The model under review builds one solid part; all positions refer to its coordinate system, in mm. Face numbers are marked on the shaded views. A direction names the side the tool comes from. Round coordinates to 2 decimals unless told otherwise and drop trailing zeros. Write each loop counter-clockwise with the first axis right and the second up, starting at its lowest first coordinate (ties: lowest second). Pieces come first, ordered by that corner, then holes. Notation, with made-up numbers: M 40.5,-32 L 84.5,-32 A10 cw 84.5,-20 Z; hole C 17.5,-37 d11. An arc over 180 degrees is marked long. One line per item, written item: value. Start each with the question number.
1) Wall thickness on probe 1 along Z at (x, y) = (-5.75, -1.95); probe 2 along X at (y, z) = (-2.05, -0.25); probe 3 along Z at (x, y) = (5.25, -2.4): over which ranges is each line inside the solid? List them lowest first.
2) Mouldability with a two-part tool opening along Z and no side actions: class the marked faces 4, 5 and 6 as +Z half, -Z half, draft (parallel to the pull), parting line (faces both ways), or undercut.
3) Take a section at A-A, the plane x = 0. Write out the cut boundary in (y, z) (1 decimal), and give its area (3 significant figures).
4) Tool access review of the marked faces 1, 2 and 3: name each direction out of +Z, -Z, +X, -X, +Y, -Y from which nothing blocks a thin tool from reaching the whole face with its end or side.
5) Take a section at C-C, the plane x = 3.5. Write out the cut boundary in (y, z) (3 decimals).
6) Take a section at D-D, the plane z = -4.25. Write out the cut boundary in (x, y) (3 decimals).
7) Take a section at B-B, the plane z = -1. Write out the cut boundary in (x, y) (3 decimals), and give its area (3 significant figures).
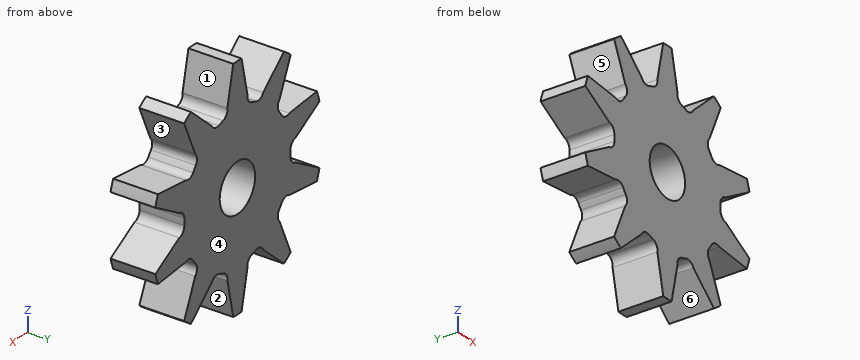
from build123d import *

# Parameters (mm, degrees)
F0_R     = 1.7145
F1_DEPTH = 3.175


with BuildPart() as f1:
    # F0 (on Front) → F1 (new body)
    with BuildSketch(Plane.XZ):
        with BuildLine():
            Line((0.97351, 5.597247), (0.402457, 8.219753))
            ThreePointArc((0.402457, 8.219753), (0, 8.2296), (-0.402457, 8.219753))
            Line((-0.402457, 8.219753), (-0.97351, 5.597247))
            ThreePointArc((-0.97351, 5.597247), (-1.052103, 5.198153), (-1.378445, 4.955349))
            ThreePointArc((-1.378445, 4.955349), (-1.589429, 4.891759), (-1.797496, 4.819191))
            ThreePointArc((-1.797496, 4.819191), (-2.204228, 4.823805), (-2.502393, 5.100483))
            Line((-2.502393, 5.100483), (-4.505855, 6.886478))
            ThreePointArc((-4.505855, 6.886478), (-4.837238, 6.657886), (-5.157044, 6.413362))
            Line((-5.157044, 6.413362), (-4.077565, 3.956053))
            ThreePointArc((-4.077565, 3.956053), (-3.906567, 3.586983), (-4.027866, 3.198732))
            ThreePointArc((-4.027866, 3.198732), (-4.161179, 3.023273), (-4.286854, 2.842266))
            ThreePointArc((-4.286854, 2.842266), (-4.618619, 2.606927), (-5.022467, 2.655508))
            Line((-5.022467, 2.655508), (-7.693084, 2.922803))
            ThreePointArc((-7.693084, 2.922803), (-7.826815, 2.543086), (-7.941816, 2.157284))
            Line((-7.941816, 2.157284), (-5.624129, 0.803781))
            ThreePointArc((-5.624129, 0.803781), (-5.268855, 0.605708), (-5.13878, 0.220308))
            ThreePointArc((-5.13878, 0.220308), (-5.1435, 0), (-5.13878, -0.220308))
            ThreePointArc((-5.13878, -0.220308), (-5.268855, -0.605708), (-5.624129, -0.803781))
            Line((-5.624129, -0.803781), (-7.941816, -2.157284))
            ThreePointArc((-7.941816, -2.157284), (-7.826815, -2.543086), (-7.693084, -2.922803))
            Line((-7.693084, -2.922803), (-5.022467, -2.655508))
            ThreePointArc((-5.022467, -2.655508), (-4.618619, -2.606927), (-4.286854, -2.842266))
            ThreePointArc((-4.286854, -2.842266), (-4.161179, -3.023273), (-4.027866, -3.198732))
            ThreePointArc((-4.027866, -3.198732), (-3.906567, -3.586983), (-4.077565, -3.956053))
            Line((-4.077565, -3.956053), (-5.157044, -6.413362))
            ThreePointArc((-5.157044, -6.413362), (-4.837238, -6.657886), (-4.505855, -6.886478))
            Line((-4.505855, -6.886478), (-2.502393, -5.100483))
            ThreePointArc((-2.502393, -5.100483), (-2.204228, -4.823805), (-1.797496, -4.819191))
            ThreePointArc((-1.797496, -4.819191), (-1.589429, -4.891759), (-1.378445, -4.955349))
            ThreePointArc((-1.378445, -4.955349), (-1.052103, -5.198153), (-0.97351, -5.597247))
            Line((-0.97351, -5.597247), (-0.402457, -8.219753))
            ThreePointArc((-0.402457, -8.219753), (0, -8.2296), (0.402457, -8.219753))
            Line((0.402457, -8.219753), (0.97351, -5.597247))
            ThreePointArc((0.97351, -5.597247), (1.052103, -5.198153), (1.378445, -4.955349))
            ThreePointArc((1.378445, -4.955349), (1.589429, -4.891759), (1.797496, -4.819191))
            ThreePointArc((1.797496, -4.819191), (2.204228, -4.823805), (2.502393, -5.100483))
            Line((2.502393, -5.100483), (4.505855, -6.886478))
            ThreePointArc((4.505855, -6.886478), (4.837238, -6.657886), (5.157044, -6.413362))
            Line((5.157044, -6.413362), (4.077565, -3.956053))
            ThreePointArc((4.077565, -3.956053), (3.906567, -3.586983), (4.027866, -3.198732))
            ThreePointArc((4.027866, -3.198732), (4.161179, -3.023273), (4.286854, -2.842266))
            ThreePointArc((4.286854, -2.842266), (4.618619, -2.606927), (5.022467, -2.655508))
            Line((5.022467, -2.655508), (7.693084, -2.922803))
            ThreePointArc((7.693084, -2.922803), (7.826815, -2.543086), (7.941816, -2.157284))
            Line((7.941816, -2.157284), (5.624129, -0.803781))
            ThreePointArc((5.624129, -0.803781), (5.268855, -0.605708), (5.13878, -0.220308))
            ThreePointArc((5.13878, -0.220308), (5.1435, 0), (5.13878, 0.220308))
            ThreePointArc((5.13878, 0.220308), (5.268855, 0.605708), (5.624129, 0.803781))
            Line((5.624129, 0.803781), (7.941816, 2.157284))
            ThreePointArc((7.941816, 2.157284), (7.826815, 2.543086), (7.693084, 2.922803))
            Line((7.693084, 2.922803), (5.022467, 2.655508))
            ThreePointArc((5.022467, 2.655508), (4.618619, 2.606927), (4.286854, 2.842266))
            ThreePointArc((4.286854, 2.842266), (4.161179, 3.023273), (4.027866, 3.198732))
            ThreePointArc((4.027866, 3.198732), (3.906567, 3.586983), (4.077565, 3.956053))
            Line((4.077565, 3.956053), (5.157044, 6.413362))
            ThreePointArc((5.157044, 6.413362), (4.837238, 6.657886), (4.505855, 6.886478))
            Line((4.505855, 6.886478), (2.502393, 5.100483))
            ThreePointArc((2.502393, 5.100483), (2.204228, 4.823805), (1.797496, 4.819191))
            ThreePointArc((1.797496, 4.819191), (1.589429, 4.891759), (1.378445, 4.955349))
            ThreePointArc((1.378445, 4.955349), (1.052103, 5.198153), (0.97351, 5.597247))
        make_face()
        Circle(F0_R, mode=Mode.SUBTRACT)
    extrude(amount=F1_DEPTH)


solid = f1.part
Checked values:
1. probe 1: z = -2.73 to -0.88, 0.88 to 2.73
1. probe 2: x = -5.14 to -1.7, 1.7 to 5.14
1. probe 3: z = -2.68 to -0.58, 0.58 to 2.68
2. face 4: draft
2. face 5: undercut
2. face 6: -Z half
3. outline: M -3.2,-8.2 L 0,-8.2 L 0,-1.7 L -3.2,-1.7 Z; M -3.2,1.7 L 0,1.7 L 0,8.2 L -3.2,8.2 Z
3. area: 41.4 mm2
4. face 1: +Z, +Y, -Y
4. face 2: -Z, +Y, -Y
4. face 3: +X, +Y, -Y
5. outline: M -3.175,-5.99 L 0,-5.99 L 0,5.99 L -3.175,5.99 Z
6. outline: M -4.207,-3.175 L 4.207,-3.175 L 4.207,0 L -4.207,0 Z
7. outline: M -5.96,-3.175 L -1.393,-3.175 L -1.393,0 L -5.96,0 Z; M 1.393,-3.175 L 5.96,-3.175 L 5.96,0 L 1.393,0 Z
7. area: 29.0 mm2
